```python
from build123d import *

# Parameters (mm, degrees)
SKETCH_1_R      = 22
EXTRUDE_1_DEPTH = 2.5


with BuildPart() as part:
    # 草圖1 → 填料-伸長1 (new, symmetric)
    with BuildSketch(Plane(origin=(0, 0, 0), x_dir=(1, 0, 0), z_dir=(0, 1, 0))):
        with BuildLine():
            ThreePointArc((0.892561983, 26.985242877), (-27, 0), (0.892561983, -26.985242877))
            ThreePointArc((0.892561983, -26.985242877), (27, 0), (0.892561983, 26.985242877))
        make_face()
        with Locations(Location((0, 0, 0), (0, 0, 270))):
            Circle(SKETCH_1_R, mode=Mode.SUBTRACT)
    extrude(amount=EXTRUDE_1_DEPTH, both=True)


solid = part.part
```
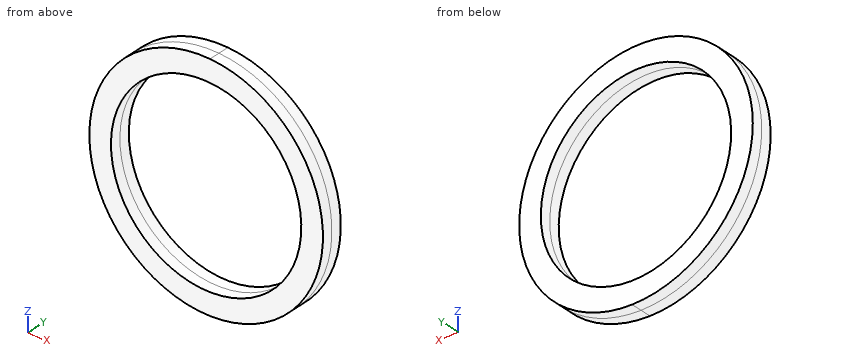
Source: CAD feature listing. Evaluate the final solid. Frame: model axes, mm. Round coordinates to 2 decimals unless told otherwise and drop trailing zeros. Loops run counter-clockwise (first coordinate to the right, second up) from the corner with the lowest first, then second, coordinate; pieces in that order, holes last. Notation, with made-up numbers: M -18.5,89 L -3.5,89 A10 ccw -3.5,104 Z; hole C 66.25,70.5 d7. An arc over 180 degrees is marked long. Put each result on its own line as item: value.
(1) Ray query, line 1 (X direction, y = 1.2, z = 0); line 2 (X direction, y = -2, z = -12.5); line 3 (Z direction, x = -10.5, y = -1.5). Return the intervals inside material, ascending. Write a range as [from, to].
Solutions:
line 1: [-27, -22], [22, 27]
line 2: [-23.93, -18.1], [18.1, 23.93]
line 3: [-24.87, -19.33], [19.33, 24.87]
(2) Section C-C, the plane y = 1.15. Return loops of the section in (x, z).
Solutions:
outline: C 0,0 d54; hole C 0,0 d44
(3) First-contact query: pin 1 (3 mm diameter, centred on y = -0.5, z = -1, fed in from -X); pin 2 (1.5 mm diameter, centred on x = -11.5, y = 0, fed in from -Z); pin 3 (1 mm diameter, centred on x = 11.5, y = -1, fed in from +Z); pin 4 (1.5 mm diameter, centred on x = 12, z = -16.5, fed in from -Y). Flat tips, straight axial feed; report the tip coordinate or a pass-through.
Solutions:
pin 1: x = -27
pin 2: z = -24.77
pin 3: z = 24.66
pin 4: through
(4) Section B-B, the plane z = 0. Return loops of the section in (x, y).
Solutions:
outline: M -27,-2.5 L -22,-2.5 L -22,2.5 L -27,2.5 Z; M 22,-2.5 L 27,-2.5 L 27,2.5 L 22,2.5 Z
(5) Section D-D, the plane x = 23.5. Return loops of the section in (y, z), and give its area (3 significant figures).
Solutions:
outline: M -2.5,-13.29 L 2.5,-13.29 L 2.5,13.29 L -2.5,13.29 Z
area: 133 mm²
(6) Section A-A, the plane x = 0. Return loops of the section in (y, z).
Solutions:
outline: M -2.5,-27 L 2.5,-27 L 2.5,-22 L -2.5,-22 Z; M -2.5,22 L 2.5,22 L 2.5,27 L -2.5,27 Z
